from build123d import *

# Parameters (mm, degrees)
BOSS_EXTRUDE1_DEPTH = 2.5
FILLET1_R           = 2
SKETCH2_R           = 1.5
CUT_EXTRUDE1_DEPTH  = 23.7981406


with BuildPart() as part:
    # Sketch1 → Boss-Extrude1 (new body)
    with BuildSketch(Plane(origin=(0, 0, 0), x_dir=(1, 0, 0), z_dir=(0, 1, 0))):
        Polygon((-1.043526837, 6.519816127), (-1.043526837, -13.480183873), (-21.043526837, -13.480183873), align=None)
    extrude(amount=BOSS_EXTRUDE1_DEPTH)

    # Fillet1
    fillet1_edges = [part.edges().sort_by_distance(p)[0] for p in [
        (-1.043526837, 1.25, -6.519816127),
        (-1.043526837, 1.25, 13.480183873),
        (-21.043526837, 1.25, 13.480183873),
    ]]
    fillet(fillet1_edges, radius=FILLET1_R)

    # Sketch2 → Cut-Extrude1 (cut, through all)
    with BuildSketch(Plane(origin=(0, 2.5, 0), x_dir=(1, 0, 0), z_dir=(0, 1, 0))):
        with Locations(Location((-4.043526837, -0.480183873, 0), (0, 0, 270))):
            Circle(SKETCH2_R)
        with Locations(Location((-4.043526837, -10.480183873, 0), (0, 0, 270))):
            Circle(SKETCH2_R)
        with Locations(Location((-14.043526837, -10.480183873, 0), (0, 0, 270))):
            Circle(SKETCH2_R)
    extrude(amount=-CUT_EXTRUDE1_DEPTH, mode=Mode.SUBTRACT)


solid = part.part
Can you work these out from the model? Positions are in its coordinate system, mm. Round coordinates to 2 decimals unless told otherwise and drop trailing zeros. Loops run counter-clockwise (first coordinate to the right, second up) from the corner with the lowest first, then second, coordinate; pieces in that order, holes last. Notation, with made-up numbers: (33, -23.5) - (70, -23.5) arc R16 ccw to (70, -11.5) - close; hole circle Ø6 at (26, 5). An arc over 180 degrees is marked (long way). Use CSV: the item, a comma, the result in double quotes. Start each with the question number.
1) If we section it at D-D on z = 5.75: Write out the boundary of the cut face in (x, y), plus the area to 3 significant figures.
2) Please list where these lines run through material, in increasing order: probe 1 along X at (y, z) = (0.3, 9.5); probe 2 along Z at (x, y) = (-3.75, 0.4); probe 3 along X at (y, z) = (0.55, 0.25). Write a range as [from, to].
3) For pin 1 Ø2.5 at (x, z) = (-4.04, 10.48) entering from +Y; pin 2 Ø6 at (x, z) = (-8, 5.5) entering from -Y, each with a flat end and sliding along its axis, tell me the tip position at first contact or that it passes through.
4) If we section it at A-A on x = -13: Write out the boundary of the cut face in (y, z).
5) If we section it at B-B on x = -5: Write out the boundary of the cut face in (y, z).
6) We'd pull the mould along Z, two halves only. Please class faces 1 (the flat face through (-8, 2.5, 7)), 2 (the cylindrical face through (-18.05, 1.27, 12.28)), 3 (the cylindrical face through (-5.51, 1.27, 0.16)): released by +Z, released by -Z, zero draft, split by the parting line, or undercut.
7) If we section it at C-C on y = 2.2: Write out the boundary of the cut face in (x, z), plus the area to 3 significant figures.
Geometry results:
1,outline,"(-13.31, 0) - (-1.04, 0) - (-1.04, 2.5) - (-13.31, 2.5) - close"
1,area,"30.7 mm2"
2,probe 1,"x = [-17.06, -15.18], [-12.91, -5.18], [-2.91, -1.04]"
2,probe 2,"z = [-3.56, -0.99], [1.95, 9.01], [11.95, 13.48]"
2,probe 3,"x = [-7.81, -5.53], [-2.56, -1.04]"
3,pin 1,"passes through"
3,pin 2,"stops at y = 0"
4,outline,"(0, 5.44) - (2.5, 5.44) - (2.5, 9.4) - (0, 9.4) - close; (0, 11.56) - (2.5, 11.56) - (2.5, 13.48) - (0, 13.48) - close"
5,outline,"(0, -2.56) - (2.5, -2.56) - (2.5, -0.68) - (0, -0.68) - close; (0, 1.64) - (2.5, 1.64) - (2.5, 9.32) - (0, 9.32) - close; (0, 11.64) - (2.5, 11.64) - (2.5, 13.48) - (0, 13.48) - close"
6,face 1,"zero draft"
6,face 2,"split by the parting line"
6,face 3,"undercut"
7,outline,"(-17.63, 10.07) - (-4.46, -3.11) arc R2 ccw to (-1.04, -1.69) - (-1.04, 11.48) arc R2 ccw to (-3.04, 13.48) - (-16.22, 13.48) arc R2 ccw to start; hole circle Ø3 at (-14.04, 10.48); hole circle Ø3 at (-4.04, 0.48); hole circle Ø3 at (-4.04, 10.48)"
7,area,"168 mm2"
